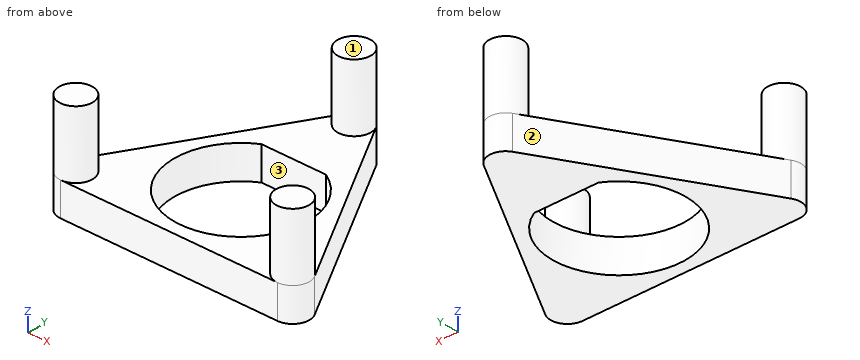
```python
from build123d import *

# Parameters (mm, degrees)
EXTRUDE_1_DEPTH     = 2
SKETCH_2_R          = 1
EXTRUDE_2_DEPTH     = 4
CUT_EXTRUDE_4_DEPTH = 5


with BuildPart() as part:
    # 草图1 → 凸台-拉伸1 (new body)
    with BuildSketch(Plane.XY):
        with BuildLine():
            Line((-7.361215932, 1.5), (-0.866025404, 12.75))
            ThreePointArc((-0.866025404, 12.75), (0, 13.25), (0.866025404, 12.75))
            Line((0.866025404, 12.75), (7.361215932, 1.5))
            ThreePointArc((7.361215932, 1.5), (7.361215932, 0.5), (6.495190528, 0))
            Line((6.495190528, 0), (-6.495190528, 0))
            ThreePointArc((-6.495190528, 0), (-7.361215932, 0.5), (-7.361215932, 1.5))
        make_face()
    extrude(amount=EXTRUDE_1_DEPTH)

    # 草图2 → 凸台-拉伸2 (add)
    with BuildSketch(Plane.XY.offset(2)):
        with Locations(Location((0, 12.25, 0), (0, 0, 150))):
            Circle(SKETCH_2_R)
        with Locations(Location((6.495190528, 1, 0), (0, 0, 270))):
            Circle(SKETCH_2_R)
        with Locations(Location((-6.495190528, 1, 0), (0, 0, 150))):
            Circle(SKETCH_2_R)
    extrude(amount=EXTRUDE_2_DEPTH)

    # 草图3 → 切除-拉伸4 (cut)
    with BuildSketch(Plane.XY.offset(2)):
        with BuildLine():
            Line((-1.936491673, 8.25), (1.936491673, 8.25))
            ThreePointArc((1.936491673, 8.25), (0, 0.75), (-1.936491673, 8.25))
        make_face()
    extrude(amount=-CUT_EXTRUDE_4_DEPTH, mode=Mode.SUBTRACT)


solid = part.part
```
For this review, take the finished solid that the model builds, in its own axes (mm). Face numbers are marked on the shaded views. Give positions to 0.01 mm unless a question says otherwise; leave off trailing zeros. Loops run counter-clockwise (first coordinate to the right, second up) from the corner with the lowest first, then second, coordinate; pieces in that order, holes last. Notation, with made-up numbers: M -15.75,84 L 40.25,84 A30 ccw 40.25,117 Z; hole C 28.25,-3 d10. An arc over 180 degrees is marked long. One line per item, written item: value. Start each with the question number.
Q1. Add section D-D (y = 4.75). Give the boundary of the cut face in (x, z).
Q2. Add section C-C (x = -1.5). Give the boundary of the cut face in (y, z), and give its area (3 significant figures).
Q3. Add section B-B (y = 1). Give the boundary of the cut face in (x, z).
Q4. Clearance check with a flat-ended pin moving along its axis: pin 1 Ø5 at (x, y) = (-1.5, 4) entering from +Z. State where the tip first meets the part, or that it passes through.
Q5. Draft analysis for pull direction X (two halves, no side actions). For the marked faces 1, 2 and 3, state which applies: released by +X, released by -X, zero draft, split by the parting line, or undercut.
Q6. For L1, parallel to Z at x = 5.25, y = 3.75; L2, parallel to X at y = 2.5, z = 0.85; L3, parallel to X at y = 3, z = 1, list the stretches that pass through material, from the lowest coordinate up.
Q7. Add section A-A (x = 0). Give the boundary of the cut face in (y, z).
Reply:
1. outline: M -5.48,0 L -4,0 L -4,2 L -5.48,2 Z; M 4,0 L 5.48,0 L 5.48,2 L 4,2 Z
2. outline: M 0,0 L 1.04,0 L 1.04,2 L 0,2 Z; M 8.25,0 L 11.65,0 L 11.65,2 L 8.25,2 Z
2. area: 8.89 mm²
3. outline: M -7.5,0 L -1.39,0 L -1.39,2 L -5.5,2 L -5.5,6 L -7.5,6 Z; M 1.39,0 L 7.5,0 L 7.5,6 L 5.5,6 L 5.5,2 L 1.39,2 Z
4. pin 1: z = 2
5. face 1: zero draft
5. face 2: released by -X
5. face 3: undercut
6. L1: 0 to 2
6. L2: -6.78 to -3.31, 3.31 to 6.78
6. L3: -6.5 to -3.6, 3.6 to 6.5
7. outline: M 0,0 L 0.75,0 L 0.75,2 L 0,2 Z; M 8.25,0 L 13.25,0 L 13.25,6 L 11.25,6 L 11.25,2 L 8.25,2 Z
